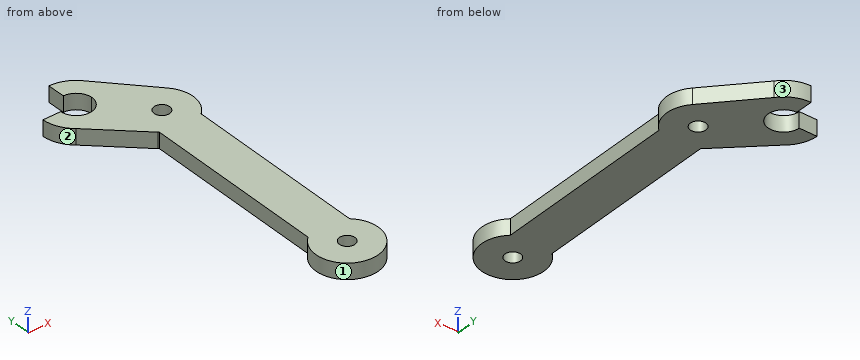
```python
from build123d import *

# Parameters (mm, degrees)
ESQUISSE1_R        = 1.5
BOSS_EXTRU_1_DEPTH = 3


with BuildPart() as part:
    # Esquisse1 → Boss.-Extru.1 (new body)
    with BuildSketch(Plane.XY):
        with BuildLine():
            Line((0, 40.527864045), (0, 4.472135955))
            ThreePointArc((0, 4.472135955), (4, -6), (8, 4.472135955))
            Line((8, 4.472135955), (8, 40.527864045))
            ThreePointArc((8, 40.527864045), (9.994318296, 44.738947964), (8.373640852, 49.107464631))
            Line((8.373640852, 49.107464631), (-0.107464631, 58.241283406))
            ThreePointArc((-0.107464631, 58.241283406), (-2.431884599, 60.07708187), (-5.329514747, 60.690941556))
            Line((-5.329514747, 60.690941556), (-5.256204762, 57.21671493))
            ThreePointArc((-5.256204762, 57.21671493), (-3.098991339, 56.376035281), (-2.168061381, 54.256204762))
            ThreePointArc((-2.168061381, 54.256204762), (-5.128571549, 51.168061381), (-8.21671493, 54.128571549))
            Line((-8.21671493, 54.128571549), (-11.690941556, 54.055261564))
            ThreePointArc((-11.690941556, 54.055261564), (-11.017535525, 51.308353115), (-9.241283406, 49.107464631))
            Line((-9.241283406, 49.107464631), (-0.163194172, 40.679373392))
            Line((-0.163194172, 40.679373392), (0, 40.527864045))
        make_face()
        with Locations((4, 0)):
            Circle(ESQUISSE1_R, mode=Mode.SUBTRACT)
        with Locations((4, 45)):
            Circle(ESQUISSE1_R, mode=Mode.SUBTRACT)
    extrude(amount=BOSS_EXTRU_1_DEPTH)


solid = part.part
```
Design review of the part built by this model. Coordinates are the model's own, in mm. Face numbers are marked on the shaded views. Round coordinates to 2 decimals unless told otherwise and drop trailing zeros. Order: outer loops, then holes, each group sorted by start corner. A loop starts at its lowest first (then second) coordinate and runs counter-clockwise, first axis right, second up. Notation, with made-up numbers: (61, 10.25) - (95, 10.25) arc R21 cw to (95, 40.25) - close; hole circle Ø5 at (-35, 56.5). An arc over 180 degrees is marked (long way). One line per question, with ' | ' between items.
Item 1: Draft analysis for pull direction Y (two halves, no side actions). For the marked faces 1, 2 and 3, state which applies: +Y half, -Y half, draft (parallel to the pull), parting line (faces both ways), or undercut.
Checks:
face 1: undercut | face 2: -Y half | face 3: +Y half
Item 2: Take a section at C-C, the plane x = 4. Write out the cut boundary in (y, z), then the cut area to 3 significant figures.
Checks:
outline: (-6, 0) - (-1.5, 0) - (-1.5, 3) - (-6, 3) - close; (1.5, 0) - (43.5, 0) - (43.5, 3) - (1.5, 3) - close; (46.5, 0) - (53.82, 0) - (53.82, 3) - (46.5, 3) - close | area: 161 mm²
Item 3: Take a section at B-B, the plane y = 0. Write out the cut boundary in (x, z), then the cut area to 3 significant figures.
Checks:
outline: (-2, 0) - (2.5, 0) - (2.5, 3) - (-2, 3) - close; (5.5, 0) - (10, 0) - (10, 3) - (5.5, 3) - close | area: 27.0 mm²
Item 4: Wall thickness on line 1 (Y direction, x = 4, z = 0.95); line 2 (Y direction, x = 3, z = 2.75); line 3 (X direction, y = 34.5, z = 2.5): over which ranges is each line inside the solid? List them lowest first. Write a range as [from, to].
Checks:
line 1: [-6, -1.5], [1.5, 43.5], [46.5, 53.82] | line 2: [-5.92, -1.12], [1.12, 43.88], [46.12, 54.89] | line 3: [0, 8]
Item 5: Take a section at A-A, the plane z = 0.8. Write out the cut boundary in (x, y) (3 decimals), then the cut area to 3 significant figures.
Checks:
outline: (-11.691, 54.055) arc R6.5 ccw to (-9.241, 49.107) - (0, 40.528) - (0, 4.472) arc R6 ccw (long way) to (8, 4.472) - (8, 40.528) arc R6 ccw to (8.374, 49.107) - (-0.107, 58.241) arc R6.5 ccw to (-5.33, 60.691) - (-5.256, 57.217) arc R3.025 cw (long way) to (-8.217, 54.129) - close; hole circle Ø3 at (4, 0); hole circle Ø3 at (4, 45) | area: 601 mm²
Item 6: Take a section at D-D, the plane y = 45. Write out the cut boundary in (x, z), then the cut area to 3 significant figures.
Checks:
outline: (-4.82, 0) - (2.5, 0) - (2.5, 3) - (-4.82, 3) - close; (5.5, 0) - (10, 0) - (10, 3) - (5.5, 3) - close | area: 35.5 mm²
Item 7: For P1, Ø1, axis at x = -2, z = 1.5, coming from the -Y side, flat-tipped, find the tip position at first contact; note if it passes through.
Checks:
P1: y = -2.4
